Read the model definition and answer for the solid it produces. Units are mm, in the model's axes. Face numbers are marked on the shaded views. A direction names the side the tool comes from. Coordinates: 2 decimals unless noted, no trailing zeros. Write each loop counter-clockwise with the first axis right and the second up, starting at its lowest first coordinate (ties: lowest second). Pieces come first, ordered by that corner, then holes. Notation, with made-up numbers: (-37.75, 54.5) -> (19.25, 54.5) arc R18 cw to (19.25, 59.5) -> close; hole circle Ø4 at (81, 16.25). An arc over 180 degrees is marked (long way). Answer as a JSON object with one key per item and string values. Group by question number.
(1) Find section B-B (x = 7.5). Give the vertices of the cut face in (y, z).
(2) Find section C-C (z = 1.7). Give the vertices of the cut face in (x, y), then the cut area to 3 significant figures.
(3) Straight lines are drawn through the part: L1, parallel to Y at x = 7.5, z = 1.15; L2, parallel to Y at x = 1.5, z = 0.5; L3, parallel to X at y = -40, z = 0.7. For each, find the intervals that lie inside material, in ascending order.
(4) Find section A-A (y = -31.5). Give the vertices of the cut face in (x, z).
(5) Which of the six approach directions +Z, -Z, +X, -X, +Y, -Y give full straight-line access (tool end or side, diameter ignored) to the marked faces 1 and 2?
(6) Find section D-D (x = 2.5). Give the vertices of the cut face in (y, z).
(7) Flat-ended cylindrical pins translate along their axes: P1, Ø1.5, axis at x = 3, z = 1.5, coming from the -Y side; P2, Ø1.8, axis at x = 7.5, y = -47.5, coming from the +Z side. Find the tip coordinate at first contact, or state that the pin passes through.
from build123d import *

# Parameters (mm, degrees)
BOSS_EXTRU_1_DEPTH      = 3
ESQUISSE3_R             = 1
ENL_V_MAT_EXTRU_1_DEPTH = 4
ESQUISSE4_R             = 1
ENL_V_MAT_EXTRU_2_DEPTH = 10


with BuildPart() as part:
    # Esquisse1 → Boss.-Extru.1 (new body)
    with BuildSketch(Plane.XY):
        with BuildLine():
            Line((0, 0), (10, 0))
            Line((10, 0), (10, -47.5))
            ThreePointArc((10, -47.5), (7.5, -50), (5, -47.5))
            Line((5, -47.5), (5, -5))
            Line((5, -5), (0, -5))
            Line((0, -5), (0, 0))
        make_face()
    extrude(amount=BOSS_EXTRU_1_DEPTH)

    # Esquisse3 → Enlèv. mat.-Extru.1 (cut)
    with BuildSketch(Plane(origin=(0, 0, 0), x_dir=(-1, 0, 0), z_dir=(0, 0, -1))):
        with Locations((-7.5, -47.5)):
            Circle(ESQUISSE3_R)
    extrude(amount=-ENL_V_MAT_EXTRU_1_DEPTH, mode=Mode.SUBTRACT)

    # Esquisse4 → Enlèv. mat.-Extru.2 (cut)
    with BuildSketch(Plane.XY.offset(3)):
        with Locations((7.5, -31.5)):
            Circle(ESQUISSE4_R)
    extrude(amount=-ENL_V_MAT_EXTRU_2_DEPTH, mode=Mode.SUBTRACT)


solid = part.part
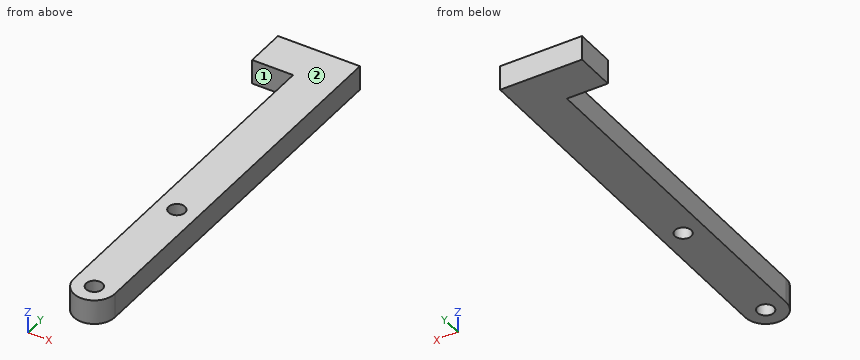
Results below:
{
 "1": {"outline": "(-50, 0) -> (-48.5, 0) -> (-48.5, 3) -> (-50, 3) -> close; (-46.5, 0) -> (-32.5, 0) -> (-32.5, 3) -> (-46.5, 3) -> close; (-30.5, 0) -> (0, 0) -> (0, 3) -> (-30.5, 3) -> close"},
 "2": {"outline": "(0, -5) -> (5, -5) -> (5, -47.5) arc R2.5 ccw to (10, -47.5) -> (10, 0) -> (0, 0) -> close; hole circle Ø2 at (7.5, -47.5); hole circle Ø2 at (7.5, -31.5)", "area": "266 mm2"},
 "3": {"L1": "y = -50 to -48.5, -46.5 to -32.5, -30.5 to 0", "L2": "y = -5 to 0", "L3": "x = 5 to 10"},
 "4": {"outline": "(5, 0) -> (6.5, 0) -> (6.5, 3) -> (5, 3) -> close; (8.5, 0) -> (10, 0) -> (10, 3) -> (8.5, 3) -> close"},
 "5": {"face 1": "+Z, -Z, -X, -Y", "face 2": "+Z, +X, -X, +Y, -Y"},
 "6": {"outline": "(-5, 0) -> (0, 0) -> (0, 3) -> (-5, 3) -> close"},
 "7": {"P1": "stops at y = -5", "P2": "passes through"}
}
